Part print with two shaded views. Sizes in mm from the minimum x, y, z corner. Give positions to 0.01 mm unless a question says otherwise; leave off trailing zeros. Write each loop counter-clockwise with the first axis right and the second up, starting at its lowest first coordinate (ties: lowest second). Pieces come first, ordered by that corner, then holes.
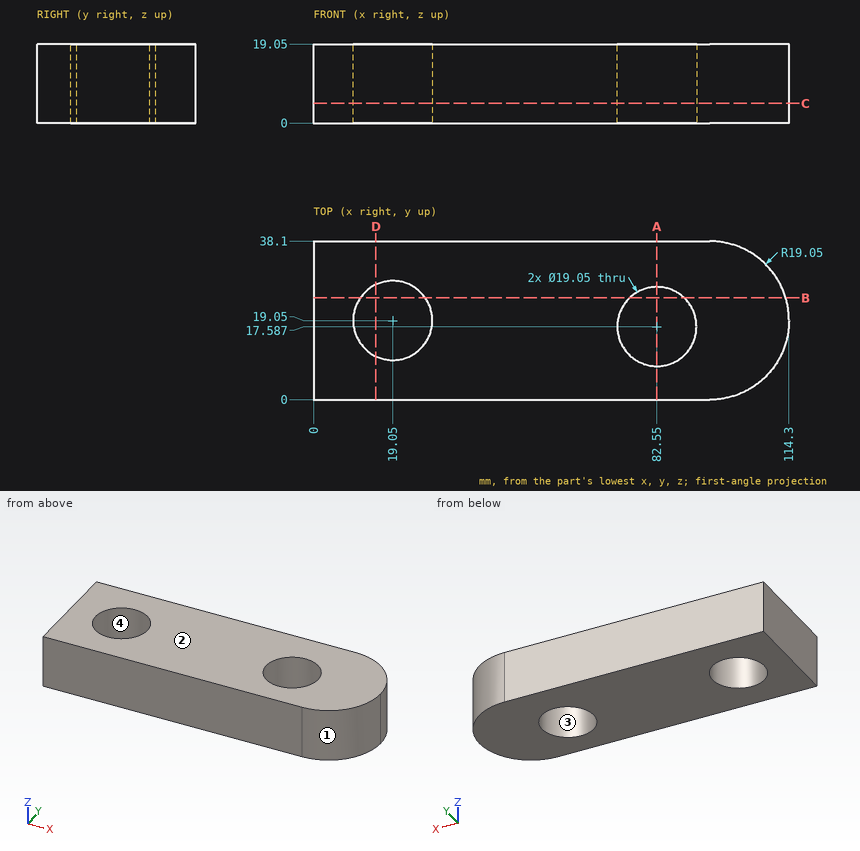
1) Saw through at B-B, the plane y = 24.5. Write the cut outline in (x, z).
Answers follow:
outline: (0, 0) - (11.24, 0) - (11.24, 19.05) - (0, 19.05) - close; (26.86, 0) - (76, 0) - (76, 19.05) - (26.86, 19.05) - close; (89.1, 0) - (113.5, 0) - (113.5, 19.05) - (89.1, 19.05) - close
2) Saw through at C-C, the plane z = 4.75. Count the separate pieces of the cut face and the enclosed holes in it, then the cut area to 3 significant figures.
Answers follow:
separate pieces: 1
enclosed holes: 2
area: 3,630 mm2
3) Pin check, flat tip, straight feed: pin 1 Ø3 at (x, z) = (100, 4.5) entering from +Y. Stop position of the tip, or through.
Answers follow:
pin 1: stops at y = 37.82
4) Wall check: L1, parallel to X at y = 15.5, z = 10.5; L2, parallel to X at y = 16, z = 8.5; L3, parallel to Y at x = 19.5, z = 11.25. Give the ranges that are in metal, low to high.
Answers follow:
L1: x = 0 to 10.21, 27.89 to 73.26, 91.84 to 113.97
L2: x = 0 to 10.03, 28.07 to 73.16, 91.94 to 114.05
L3: y = 0 to 9.54, 28.56 to 38.1
5) Saw through at A-A, the plane x = 82.55. Write the cut outline in (y, z), then the cut area to 3 significant figures.
Answers follow:
outline: (0, 0) - (8.06, 0) - (8.06, 19.05) - (0, 19.05) - close; (27.11, 0) - (38.1, 0) - (38.1, 19.05) - (27.11, 19.05) - close
area: 363 mm2
6) Two-plate mould, pull along Y, no slides. Class the marked faces 1, 2, 3 and 4: +Y half, -Y half, draft (parallel to the pull), parting line (faces both ways), or undercut.
Answers follow:
face 1: -Y half
face 2: draft
face 3: undercut
face 4: undercut
7) Saw through at D-D, the plane x = 15. Write the cut outline in (y, z), then the cut area to 3 significant figures.
Answers follow:
outline: (0, 0) - (10.43, 0) - (10.43, 19.05) - (0, 19.05) - close; (27.67, 0) - (38.1, 0) - (38.1, 19.05) - (27.67, 19.05) - close
area: 397 mm2
